CAD build for the part. Positions are in the model's coordinates, mm. Face numbers are marked on the shaded views. Round coordinates to 2 decimals unless told otherwise and drop trailing zeros. Write each loop counter-clockwise with the first axis right and the second up, starting at its lowest first coordinate (ties: lowest second). Pieces come first, ordered by that corner, then holes. Notation, with made-up numbers: (15, 58.5) - (24, 58.5) arc R25 ccw to (24, 82.5) - close; hole circle Ø7 at (-12, -12.5). An arc over 180 degrees is marked (long way). Answer in a Markdown table with one row per item.
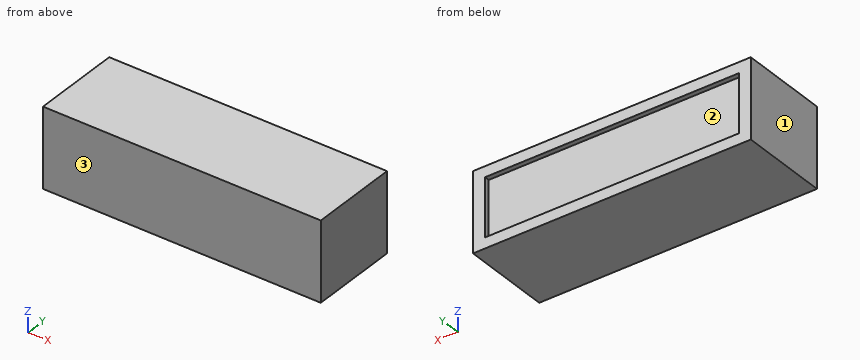
```python
from build123d import *

# Parameters (mm, degrees)
SKETCH1_W           = 28
SKETCH1_H           = 9
BOSS_EXTRUDE1_DEPTH = 8
CUT_EXTRUDE1_DEPTH  = 0.5


with BuildPart() as part:
    # Sketch1 → Boss-Extrude1 (new body)
    with BuildSketch(Plane.XY):
        with Locations((14, 4.5)):
            Rectangle(SKETCH1_W, SKETCH1_H)
    extrude(amount=BOSS_EXTRUDE1_DEPTH)

    # Sketch2 → Cut-Extrude1 (cut)
    with BuildSketch(Plane(origin=(0, 9, 0), x_dir=(1, 0, 0), z_dir=(0, 1, 0))):
        Polygon((14, -1.074899), (1.215291321, -1.074899), (1.215291321, -4), (1.215291321, -6.925101), (26.784708679, -6.925101), (26.784708679, -1.074899), align=None)
    extrude(amount=-CUT_EXTRUDE1_DEPTH, mode=Mode.SUBTRACT)


solid = part.part
```
Q1. Saw through at B-B on z = 1.5. List the corners of the cut face in (x, y).
Computed:
| item | result |
|---|---|
| outline | (0, 0) - (28, 0) - (28, 9) - (26.78, 9) - (26.78, 8.5) - (1.22, 8.5) - (1.22, 9) - (0, 9) - close |
Q2. Flat gauge pin, fed straight in: pin 1 (1.5 mm diameter, centred on x = 4, z = 2, fed in from +Y). Where does the tip first touch, or does it go through?
Computed:
| item | result |
|---|---|
| pin 1 | stops at y = 8.5 |
Q3. Saw through at A-A on x = 18. List the corners of the cut face in (y, z), then the cut area to 3 significant figures.
Computed:
| item | result |
|---|---|
| outline | (0, 0) - (9, 0) - (9, 1.07) - (8.5, 1.07) - (8.5, 6.93) - (9, 6.93) - (9, 8) - (0, 8) - close |
| area | 69.1 mm2 |
Q4. Drill centre line: line 1 (Y direction, x = 21, z = 3.25). Where is it in solid material? Low to high.
Computed:
| item | result |
|---|---|
| line 1 | y = 0 to 8.5 |
Q5. Pull direction X, two halves, no side cores. Call the marked faces 1, 2 and 3: released by +X, released by -X, zero draft, split by the parting line, or undercut.
Computed:
| item | result |
|---|---|
| face 1 | released by -X |
| face 2 | undercut |
| face 3 | zero draft |
